Solid Edge part; units mm, degrees
sketch "Sketch1" plane through (0, 0, 0) normal (0, 0, 1) x (1, 0, 0)
  line L0 (3.8532, 3.1931) -> (5.8532, 3.1931)
  line L1 (5.8532, 3.1931) -> (5.8532, -16.8069)
  line L2 (5.8532, -16.8069) -> (6.8532, -16.8069)
  line L3 (6.8532, 4.1931) -> (6.8532, -16.8069)
  line L4 (3.8532, 4.1931) -> (6.8532, 4.1931)
  line L5 (3.8532, 4.1931) -> (3.8532, 3.1931)
extrude "Protrusion1" add sketch "Sketch1" against normal blind 20
Check sheet for the modelled part. Datum: model origin and axes. Units: mm. A direction names the side the tool comes from. Coordinates: 2 decimals unless noted, no trailing zeros. Loops run counter-clockwise (first coordinate to the right, second up) from the corner with the lowest first, then second, coordinate; pieces in that order, holes last. Notation, with made-up numbers: (38.25, 18) -> (55.25, 18) arc R3 ccw to (55.25, 23) -> close; hole circle Ø4 at (-11, 41.5). An arc over 180 degrees is marked (long way). Answer in a Markdown table with one row per item.
1. Sectioned sample at B-B, the plane x = 5.1. Record the boundary of the cut face in (y, z), then the cut area to 3 significant figures.
Check values:
| item | result |
|---|---|
| outline | (3.19, -20) -> (4.19, -20) -> (4.19, 0) -> (3.19, 0) -> close |
| area | 20.0 mm2 |
2. Material ranges on line 1 along Y through (x, z) = (5.1, -15.5); line 2 along X through (y, z) = (-7.75, -14), recorded low to high. Write a range as [from, to].
Check values:
| item | result |
|---|---|
| line 1 | y = [3.19, 4.19] |
| line 2 | x = [5.85, 6.85] |
3. Sectioned sample at C-C, the plane y = -5.75. Record the boundary of the cut face in (x, z).
Check values:
| item | result |
|---|---|
| outline | (5.85, -20) -> (6.85, -20) -> (6.85, 0) -> (5.85, 0) -> close |
4. Access from +Z, -Z, +X, -X, +Y, -Y to the whole of each face (thin tool, end or side, straight path). Record for faces 1 (the face through (5.853, -7, -10)), 2 (the face through (6.853, -6, -10)).
Check values:
| item | result |
|---|---|
| face 1 | +Z, -Z, -X, -Y |
| face 2 | +Z, -Z, +X, +Y, -Y |
5. Sectioned sample at A-A, the plane z = -7. Record the boundary of the cut face in (x, y).
Check values:
| item | result |
|---|---|
| outline | (3.85, 3.19) -> (5.85, 3.19) -> (5.85, -16.81) -> (6.85, -16.81) -> (6.85, 4.19) -> (3.85, 4.19) -> close |
6. Go/stop test with flat-tipped pins: pin 1 (1.6 mm diameter, centred on x = 4.5, z = -5.5, fed in from -Y); pin 2 (10 mm diameter, centred on y = -3.5, z = -5.5, fed in from -X). Record where each tip stops, or that it passes through.
Check values:
| item | result |
|---|---|
| pin 1 | stops at y = 3.19 |
| pin 2 | stops at x = 5.85 |
